Check sheet for the drawn part. Datum: minimum x, y, z corner. Units: mm. A direction names the side the tool comes from. Coordinates: 2 decimals unless noted, no trailing zeros. Write each loop counter-clockwise with the first axis right and the second up, starting at its lowest first coordinate (ties: lowest second). Pieces come first, ordered by that corner, then holes. Notation, with made-up numbers: (-8.5, -5) - (4.5, -5) arc R11 ccw to (4.5, 13) - close; hole circle Ø4 at (-38.75, 79.25). An arc over 180 degrees is marked (long way). Use CSV: the item, a comma, the result in double quotes. Start each with the question number.
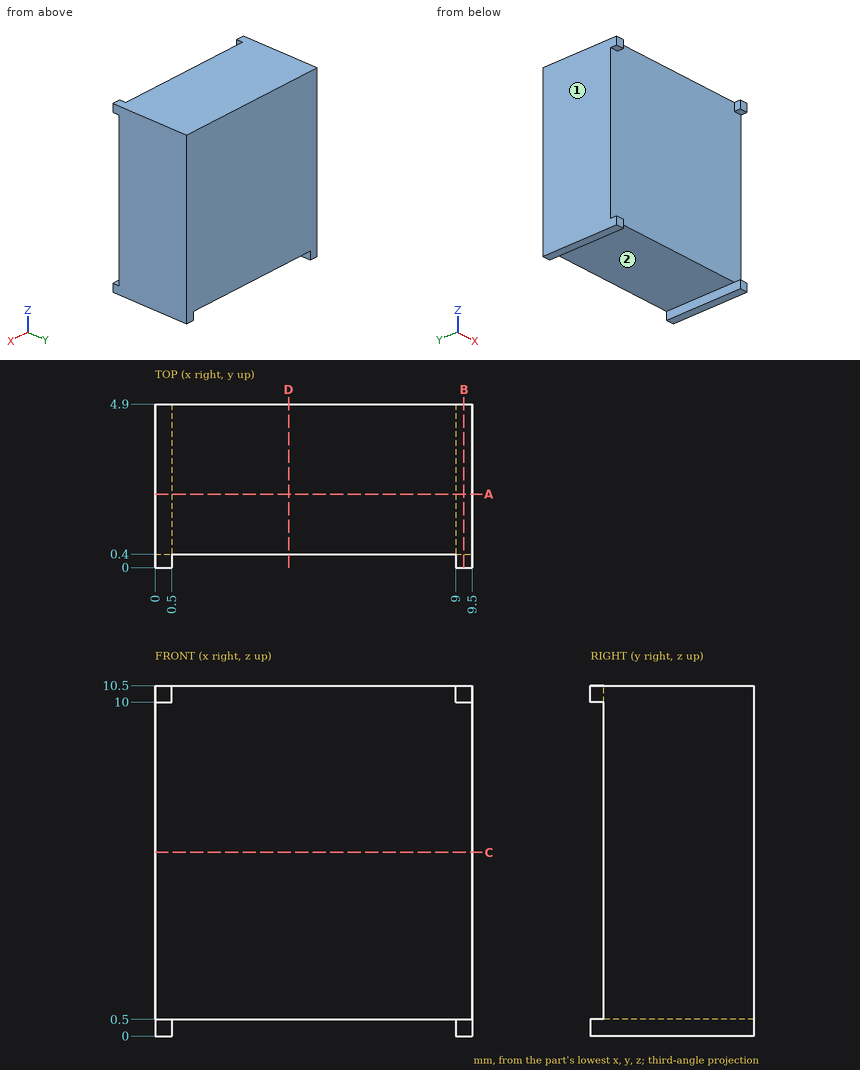
Q1. Cross-section at D-D (x = 4). Record the cut outline in (y, z).
Q2. Tool access check on the marked faces 1 and 2. Record the directions out of +Z, -Z, +X, -X, +Y, -Y that give a thin tool (end or side, any length) a straight path to the whole face; none if there is none.
Q3. Cross-section at C-C (z = 5.5). Record the cut outline in (x, y), plus the area to 4 significant figures.
Q4. Scan lines: line 1 along Y through (x, z) = (4, 8); line 2 along Z through (x, y) = (3.25, 1.7). Record each from-to range of solid material in increasing order. Write a range as from..to.
Q5. Cross-section at A-A (y = 2.2). Record the cut outline in (x, z), plus the area to 3 significant figures.
Q6. Cross-section at B-B (x = 9.25). Record the cut outline in (y, z).
Q7. Gauge pin test, flat end, axial feed: pin 1 (3 mm diameter, centred on x = 3, z = 2.5, fed in from -Y). Record the tip position at first contact, or that the pin passes through.
Reply:
1,outline,"(0.4, 0.5) - (4.9, 0.5) - (4.9, 10.5) - (0.4, 10.5) - close"
2,face 1,"+Z, -Z, -X, +Y, -Y"
2,face 2,"-Z, +Y, -Y"
3,outline,"(0, 0.4) - (9.5, 0.4) - (9.5, 4.9) - (0, 4.9) - close"
3,area,"42.75 mm^2"
4,line 1,"0.4..4.9"
4,line 2,"0.5..10.5"
5,outline,"(0, 0) - (0.5, 0) - (0.5, 0.5) - (9, 0.5) - (9, 0) - (9.5, 0) - (9.5, 10.5) - (0, 10.5) - close"
5,area,"95.5 mm^2"
6,outline,"(0, 0) - (4.9, 0) - (4.9, 10.5) - (0, 10.5) - (0, 10) - (0.4, 10) - (0.4, 0.5) - (0, 0.5) - close"
7,pin 1,"y = 0.4"
